Geometry check sheet. Reference: drawing and pictorial views, mm from the part's lowest x, y, z. Coordinates: 2 decimals unless noted, no trailing zeros. Loops run counter-clockwise (first coordinate to the right, second up) from the corner with the lowest first, then second, coordinate; pieces in that order, holes last. Notation, with made-up numbers: (-24.5, 15) - (-15.5, 15) arc R9 cw to (-15.5, 32) - close; hole circle Ø8 at (-10.75, 35). An arc over 180 degrees is marked (long way). Use a Markdown table: item, result. Add a question column.
1) Sectioned sample at B-B, the plane x = 55. Enter the section's corners in (y, z).
2) Thickness scan on line 1 (X direction, y = 119, z = 29.5); line 2 (Y direction, x = 50, z = 28.5) (1 decimal); line 3 (Y direction, x = 17, z = 24.5) (1 decimal). Record the ranges inside material, lowest first.
3) Go/stop test with flat-tipped pins: P1, Ø1.5, axis at x = 40.5, z = 26.5, coming from the +Y side; P2, Ø1.5, axis at x = 23, z = 16, coming from the +Y side; P3, Ø6, axis at x = 9.5, z = 33, coming from the -Y side (1 decimal). Record where each tip stops, or that it passes through.
4) Sectioned sample at A-A, the plane z = 26.5. Enter the section's corners in (x, y), then the cut area to 3 significant figures.
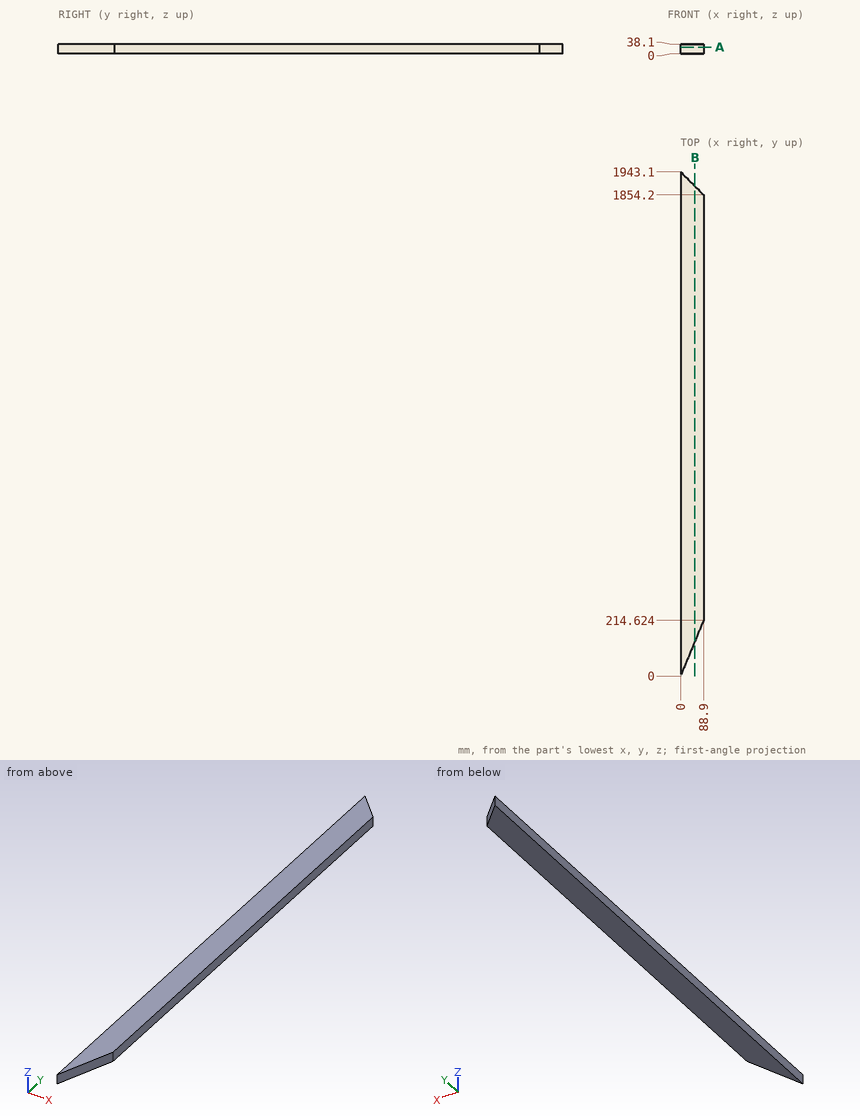
Solved:
| question | item | result |
|---|---|---|
| 1 | outline | (132.78, 0) - (1888.1, 0) - (1888.1, 38.1) - (132.78, 38.1) - close |
| 2 | line 1 | x = 0 to 49.29 |
| 2 | line 2 | y = 120.7 to 1893.1 |
| 2 | line 3 | y = 41 to 1926.1 |
| 3 | P1 | stops at y = 1903.35 |
| 3 | P2 | stops at y = 1920.85 |
| 3 | P3 | stops at y = 15.7 |
| 4 | outline | (0, 0) - (88.9, 214.62) - (88.9, 1854.2) - (0, 1943.1) - close |
| 4 | area | 159,000 mm2 |
